from build123d import *

# Parameters (mm, degrees)
F0_W      = 60
F0_H      = 115
F1_DEPTH  = 12
F2_W      = 60
F2_H      = 12
F3_DEPTH  = 48
F4_W      = 20
F4_H      = 50
F5_DEPTH  = 48
F6_R      = 12.5
F7_DEPTH  = 20.001
F9_DEPTH  = 20.001
F11_DEPTH = 12.001


with BuildPart() as f1:
    # F0 (on Top) → F1 (new body)
    with BuildSketch(Plane.XY):
        Rectangle(F0_W, F0_H)
    extrude(amount=F1_DEPTH)

    # F2 (on face) → F3 (join)
    with BuildSketch(Plane.XY.offset(12)):
        with Locations((0, 51.5)):
            Rectangle(F2_W, F2_H)
    extrude(amount=F3_DEPTH)

    # F4 (on face) → F5 (join)
    with BuildSketch(Plane.XY.offset(12)):
        with Locations((-20, -32.5)):
            Rectangle(F4_W, F4_H)
    extrude(amount=F5_DEPTH)

    # F6 (on face) → F7 (cut, through all)
    with BuildSketch(Plane.YZ.offset(-10)):
        with Locations((-32.5, 35)):
            Circle(F6_R)
    extrude(amount=-F7_DEPTH, mode=Mode.SUBTRACT)

    # F8 (on face) → F9 (cut, through all)
    with BuildSketch(Plane.YZ.offset(-10)):
        with BuildLine():
            ThreePointArc((-57.5, 35), (-50.17767, 52.67767), (-32.5, 60))
            Line((-32.5, 60), (-57.5, 60))
            Line((-57.5, 60), (-57.5, 35))
        make_face()
        with BuildLine():
            ThreePointArc((-32.5, 60), (-14.82233, 52.67767), (-7.5, 35))
            Line((-7.5, 35), (-7.5, 60))
            Line((-7.5, 60), (-32.5, 60))
        make_face()
    extrude(amount=-F9_DEPTH, mode=Mode.SUBTRACT)

    # F10 (on face) → F11 (cut, through all)
    with BuildSketch(Plane.XY.offset(12)):
        Polygon((30, 45.5), (-10, -57.5), (30, -57.5), align=None)
    extrude(amount=-F11_DEPTH, mode=Mode.SUBTRACT)


solid = f1.part
Design review of the part built by this model. Coordinates are the model's own, in mm. A direction names the side the tool comes from. Coordinates: 2 decimals unless noted, no trailing zeros. Order: outer loops, then holes, each group sorted by start corner. A loop starts at its lowest first (then second) coordinate and runs counter-clockwise, first axis right, second up. Notation, with made-up numbers: (36, 51) -> (61, 51) arc R22 cw to (61, 65) -> close; hole circle Ø3 at (-15, 29). An arc over 180 degrees is marked (long way). One line per item, written item: value.
1) We need section D-D, the plane x = 24. Give the boundary of the cut face in (y, z), then the cut area to 3 significant figures.
Output values:
outline: (30.05, 0) -> (57.5, 0) -> (57.5, 60) -> (45.5, 60) -> (45.5, 12) -> (30.05, 12) -> close
area: 905 mm2
2) Machinability: for faces 1 (the face through (10.28, -5.28, 6.08)), 2 (the face through (-10, -44, 41)), 3 (the face through (-20, -7.5, 23)), which of the approach directions +Z, -Z, +X, -X, +Y, -Y give a long, thin tool a straight path to every point of the face, cutting with its end or side? Answer none if there is none.
Output values:
face 1: +Z, -Z, +X, -Y
face 2: +Z, +X, -Y
face 3: +Z, +X, -X
3) We need section B-B, the plane x = -20. Give the boundary of the cut face in (y, z).
Output values:
outline: (-57.5, 0) -> (57.5, 0) -> (57.5, 60) -> (45.5, 60) -> (45.5, 12) -> (-7.5, 12) -> (-7.5, 35) arc R25 ccw to (-32.5, 60) arc R25 ccw to (-57.5, 35) -> close; hole circle Ø25 at (-32.5, 35)
4) To check wall thickness, follow probe 1 along Z at (x, y) = (-25, -32.5); probe 2 along Y at (x, z) = (11, 50); probe 3 along X at (y, z) = (-47, 41.5). State the ranges of each line that lie inside material, in increasing order. Write a range as [from, to].
Output values:
probe 1: z = [0, 22.5], [47.5, 60]
probe 2: y = [45.5, 57.5]
probe 3: x = [-30, -10]
5) Draft analysis for pull direction Y (two halves, no side actions). For faces 4 (the face through (30, 51, 30)), 5 (the face through (0, 45.5, 36)), 6 (the face through (0, 57.5, 30)), state which applies: +Y half, -Y half, draft (parallel to the pull), parting line (faces both ways), or undercut.
Output values:
face 4: draft
face 5: undercut
face 6: +Y half
6) Clearance check with a flat-ended pin moving along its axis: P1, Ø24, axis at x = 5, z = 29.5, coming from the -Y side. State where the tip first meets the part, or that it passes through.
Output values:
P1: stops at y = 45.5
7) We need section C-C, the plane z = 32.5. Give the boundary of the cut face in (x, y), then the cut area to 3 significant figures.
Output values:
outline: (-30, -57.5) -> (-10, -57.5) -> (-10, -44.75) -> (-30, -44.75) -> close; (-30, -20.25) -> (-10, -20.25) -> (-10, -7.5) -> (-30, -7.5) -> close; (-30, 45.5) -> (30, 45.5) -> (30, 57.5) -> (-30, 57.5) -> close
area: 1,230 mm2
8) We need section A-A, the plane z = 14.5. Give the boundary of the cut face in (x, y), then the cut area to 3 significant figures.
Output values:
outline: (-30, -57.5) -> (-10, -57.5) -> (-10, -7.5) -> (-30, -7.5) -> close; (-30, 45.5) -> (30, 45.5) -> (30, 57.5) -> (-30, 57.5) -> close
area: 1,720 mm2
